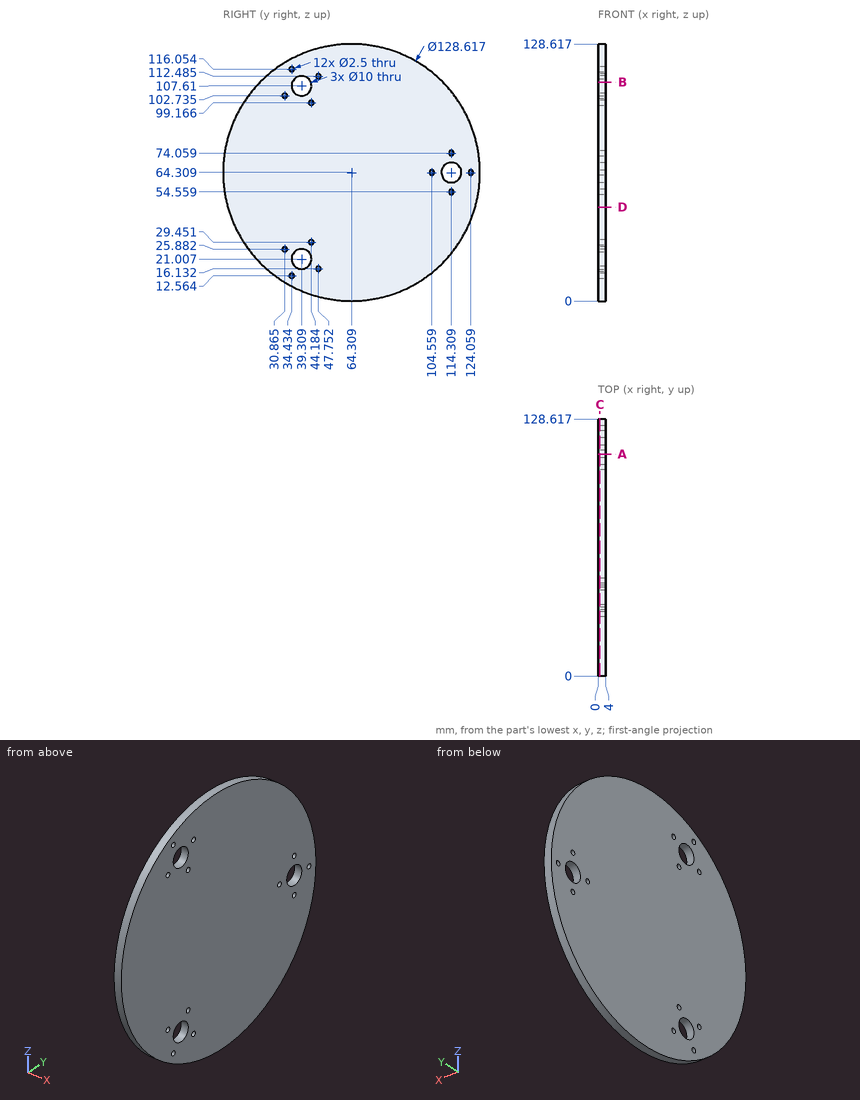
Part print with two shaded views. Sizes in mm from the minimum x, y, z corner. Round coordinates to 2 decimals unless told otherwise and drop trailing zeros. Write each loop counter-clockwise with the first axis right and the second up, starting at its lowest first coordinate (ties: lowest second). Pieces come first, ordered by that corner, then holes. Notation, with made-up numbers: (65.25, 74) -> (101.25, 74) arc R18 ccw to (101.25, 88) -> close; hole circle Ø10 at (7, 2.25). An arc over 180 degrees is marked (long way). Use one line per item in the form item = value.
Q1. Band-saw the part on A-A, the plane y = 111. Write the cut outline in (x, z).
Conclusion:
outline = (0, 20.09) -> (4, 20.09) -> (4, 60.56) -> (0, 60.56) -> close; (0, 68.06) -> (4, 68.06) -> (4, 108.53) -> (0, 108.53) -> close
Q2. Band-saw the part on C-C, the plane x = 0.9. State how many separate pieces and enclosed holes the cut face has, then the cut area to 3 significant figures.
Conclusion:
separate_pieces = 1
enclosed_holes = 15
area = 12,700 mm²
Q3. Drill centre lines: L1, parallel to Z at x = 0.35, y = 38 (1 decimal); L2, parallel to Y at x = 1.7, z = 103 (1 decimal); L3, parallel to Y at x = 0.7, z = 13 (1 decimal). Where is each one in solid material? Low to high.
Conclusion:
L1 = 5.6 to 16.2, 25.8 to 102.8, 112.4 to 123
L2 = 12.9 to 29.6, 32.1 to 37.4, 41.2 to 115.7
L3 = 25.5 to 33.3, 35.6 to 103.1
Q4. Band-saw the part on B-B, the plane z = 109.5. Write the cut outline in (x, y) (1 decimal).
Conclusion:
outline = (0, 18.6) -> (4, 18.6) -> (4, 34.7) -> (0, 34.7) -> close; (0, 43.9) -> (4, 43.9) -> (4, 110.1) -> (0, 110.1) -> close
Q5. Band-saw the part on D-D, the plane z = 47. Write the cut outline in (x, y).
Conclusion:
outline = (0, 2.37) -> (4, 2.37) -> (4, 126.24) -> (0, 126.24) -> close
Q6. Drop a flat-ended pin along its axis: P1, Ø2, axis at x = 1, z = 68.5, coming from the -Y side. Give the stop position or say it passes through.
Conclusion:
P1 = 0.08
